from build123d import *

# Parameters (mm, degrees)
SKETCH_R      = 8
PAD_DEPTH     = 5
SKETCH001_R   = 10
SKETCH001_R_2 = 6
PAD001_DEPTH  = 2


with BuildPart() as part:
    # Sketch → Pad (new body)
    with BuildSketch(Plane.XY):
        with BuildLine():
            ThreePointArc((-2.142857, -9.76771), (10, 0), (-2.142857, 9.76771))
            Line((-28.857143, 3.907084), (-2.142857, 9.76771))
            ThreePointArc((-28.857143, 3.907084), (-32, 0), (-28.857143, -3.907084))
            Line((-2.142857, -9.76771), (-28.857143, -3.907084))
        make_face()
        Circle(SKETCH_R, mode=Mode.SUBTRACT)
    extrude(amount=PAD_DEPTH)

    # Sketch001 (on Face7 of Pad) → Pad001 (join)
    with BuildSketch(Plane.XY.offset(5)):
        Circle(SKETCH001_R)
        Circle(SKETCH001_R_2, mode=Mode.SUBTRACT)
    extrude(amount=PAD001_DEPTH)


solid = part.part
Work out the finished part from the listing and answer in its coordinate system (mm). A direction names the side the tool comes from. Give positions to 0.01 mm unless a question says otherwise; leave off trailing zeros. Order: outer loops, then holes, each group sorted by start corner. A loop starts at its lowest first (then second) coordinate and runs counter-clockwise, first axis right, second up. Notation, with made-up numbers: (15.25, 42) -> (56.25, 42) arc R17 cw to (56.25, 66) -> close; hole circle Ø7 at (38.25, -14.75). An arc over 180 degrees is marked (long way). Answer as a JSON object with one key per item and string values. Group by question number.
1. Section C-C on z = 0.5 is taken. Determine the outline of the cut face in (x, y), plus the area to 3 significant figures.
2. A tool of negligible diameter and unlimited length cuts with its end or side. For faces 1 (the flat face through (-15.687, 6.796, 2.465)), 2 (the cylindrical face through (-1.73, -7.81, 2.46)), from which of +Z, -Z, +X, -X, +Y, -Y can it reach the whole face along a straight path? Write none if from no direction.
3. A flat-ended cylindrical pin translates along its axis: pin 1 Ø3 at (y, z) = (-7.5, 1.5) entering from +X. Find the tip coordinate at first contact, or state that the pin passes through.
4. Section A-A on y = 0 is taken. Determine the outline of the cut face in (x, z), plus the area to 3 significant figures.
5. Consider line 1 along Y through (x, z) = (0, 2.4); line 2 along Y through (x, z) = (0, 6.25); line 3 along X through (y, z) = (-0.5, 1). Determine where each line is inside the solid, lowest interval first. Write a range as [from, to].
6. The mould has two halves that part along X. Classify faces 3 (the flat face through (-11, 0, 0)), 4 (the cylindrical face through (-32, 0, 2)), 5 (the cylindrical face through (-6, 0, 6)): released by +X, released by -X, zero draft, split by the parting line, or undercut.
7. Section D-D on x = 7.5 is taken. Determine the outline of the cut face in (y, z).
8. Section B-B on x = 0 is taken. Determine the outline of the cut face in (y, z).
Result sheet:
{
 "1": {"outline": "(-28.86, -3.91) -> (-2.14, -9.77) arc R10 ccw (long way) to (-2.14, 9.77) -> (-28.86, 3.91) arc R4 ccw to start; hole circle Ø16 at (0, 0)", "area": "382 mm^2"},
 "2": {"face 1": "+Z, -Z, -X, +Y", "face 2": "-Z"},
 "3": {"pin 1": "stops at x = 8"},
 "4": {"outline": "(-32, 0) -> (-8, 0) -> (-8, 5) -> (-6, 5) -> (-6, 7) -> (-10, 7) -> (-10, 5) -> (-32, 5) -> close; (6, 5) -> (8, 5) -> (8, 0) -> (10, 0) -> (10, 7) -> (6, 7) -> close", "area": "146 mm^2"},
 "5": {"line 1": "y = [-10, -8], [8, 10]", "line 2": "y = [-10, -6], [6, 10]", "line 3": "x = [-31.97, -7.98], [7.98, 9.99]"},
 "6": {"face 3": "zero draft", "face 4": "released by -X", "face 5": "undercut"},
 "7": {"outline": "(-6.61, 0) -> (-2.78, 0) -> (-2.78, 5) -> (2.78, 5) -> (2.78, 0) -> (6.61, 0) -> (6.61, 7) -> (-6.61, 7) -> close"},
 "8": {"outline": "(-10, 0) -> (-8, 0) -> (-8, 5) -> (-6, 5) -> (-6, 7) -> (-10, 7) -> close; (6, 5) -> (8, 5) -> (8, 0) -> (10, 0) -> (10, 7) -> (6, 7) -> close"}
}
